from build123d import *

# Parameters (mm, degrees)
F2_R     = 2.5
F3_DEPTH = 25
F4_R     = 5
F5_DEPTH = 29


with BuildPart() as f1:
    # F0 (on Front) → F1 (revolve)
    with BuildSketch(Plane.XZ):
        with BuildLine():
            Line((0, 29.563617), (0, 0))
            Line((0, 0), (35, 0))
            Line((35, 0), (35, 9.045376))
            ThreePointArc((35, 9.045376), (34.12132, 11.166697), (32, 12.045376))
            Line((32, 12.045376), (15.753854, 12.045376))
            Line((15.753854, 12.045376), (13.664301, 22.045376))
            ThreePointArc((13.664301, 22.045376), (10.182308, 27.760598), (3.875714, 30))
            Line((3.875714, 30), (3.702194, 30))
            add(Edge.make_bspline(
                [(3.702194, 30), (2.872247, 30.008527), (3.357668, 29.526608), (0, 29.563617)],
                knots=[0, 0, 0, 0, 3.727824, 3.727824, 3.727824, 3.727824], degree=3))
        make_face()
    revolve(axis=Axis((0, 0, 14.781808), (0, 0, 1)))

    # F2 (on face) → F3 (cut)
    with BuildSketch(Plane.XY.offset(12.045376)):
        with Locations((0, 27.485492)):
            Circle(F2_R)
        with Locations((23.803134, -13.742746)):
            Circle(F2_R)
        with Locations((-23.803134, -13.742746)):
            Circle(F2_R)
    extrude(amount=-F3_DEPTH, mode=Mode.SUBTRACT)

    # F4 (on face) → F5 (join)
    with BuildSketch(Plane(origin=(0, 0, 0), x_dir=(1, 0, 0), z_dir=(0, 0, -1))):
        Circle(F4_R)
    extrude(amount=-F5_DEPTH)


solid = f1.part
For this review, take the finished solid that the model builds, in its own axes (mm). Round coordinates to 2 decimals unless told otherwise and drop trailing zeros. Loops run counter-clockwise (first coordinate to the right, second up) from the corner with the lowest first, then second, coordinate; pieces in that order, holes last. Notation, with made-up numbers: (88.25, 49.25) - (142.25, 49.25) arc R22 ccw to (142.25, 59.25) - close; hole circle Ø9 at (83, 58). An arc over 180 degrees is marked (long way). Answer as CSV lines item,"result".
(1) Consider section A-A on z = 19. Give the boundary of the cut face in (x, y).
Checked values:
outline,"circle Ø28.6 at (0, 0)"
(2) Mouldability with a two-part tool opening along Y and no side actions: class faces 1 (the face through (7, 15, 12.045)), 2 (the face through (-28, -21, 5)), 3 (the face through (-0.542, 25.045, 6.107)) as +Y half, -Y half, draft (parallel to the pull), parting line (faces both ways), or undercut.
Checked values:
face 1,"draft"
face 2,"parting line"
face 3,"undercut"
(3) Wall thickness on line 1 (Y direction, x = 0, z = 3); line 2 (Z direction, x = -13.5, y = 17.5); line 3 (Z direction, x = -5.5, y = -4): over which ranges is each line inside the solid? List them lowest first.
Checked values:
line 1,"y = -35 to 24.99, 29.99 to 35"
line 2,"z = 0 to 12.05"
line 3,"z = 0 to 29.56"
(4) Insertion check: P1, Ø3, axis at x = -5, y = -9, coming from the +Z side; P2, Ø2, axis at x = -11.5, z = 3.5, coming from the -Y side; P3, Ø6, axis at x = 23.8, y = -13.74, coming from the +Z side. Each pin has a flat end and moves straight along its axis. Give the tip position at first contact, or say it passes through.
Checked values:
P1,"stops at z = 28.71"
P2,"stops at y = -33.39"
P3,"stops at z = 12.05"
